```python
from build123d import *

# Parameters (mm, degrees)
F0_W      = 121.92
F0_H      = 71.12
F1_DEPTH  = 35.56
F2_W      = 3.81
F2_H      = 3.81
F3_DEPTH  = 12.7
F4_W      = 69.85
F4_H      = 47.625
F5_DEPTH  = 15.24
F6_W      = 27.94
F6_H      = 6.35
F7_DEPTH  = 71.12
F8_W      = 15.24
F8_H      = 6.35
F9_DEPTH  = 121.92
F10_W     = 27.94
F10_H     = 15.24
F11_DEPTH = 15.24
F12_DEPTH = 35.561
F13_W     = 40.005
F13_H     = 6.6675
F14_DEPTH = 35.561
F15_W     = 40.005
F15_H     = 15.24
F16_DEPTH = 4.2690588161
F17_W     = 40.005
F17_H     = 15.24
F18_DEPTH = 4.0254006162
F19_W     = 20.955
F19_H     = 14.605
F20_DEPTH = 25.4
F21_W     = 14.605
F21_H     = 15.24
F22_DEPTH = 17.6893454045
F23_W     = 14.605
F23_H     = 15.24
F24_DEPTH = 16.1260850728
F25_W     = 20.955
F25_H     = 15.24
F26_DEPTH = 12.7
F27_W     = 6.6675
F27_H     = 15.24
F28_DEPTH = 25.4
F29_W     = 6.6675
F29_H     = 15.24
F30_DEPTH = 25.4
F31_W     = 20.955
F31_H     = 15.24
F32_DEPTH = 12.7


with BuildPart() as f1:
    # F0 (on Top) → F1 (new body)
    with BuildSketch(Plane.XY):
        Rectangle(F0_W, F0_H)
    extrude(amount=F1_DEPTH)

    # F2 (on Top) → F3 (cut)
    with BuildSketch(Plane.XY):
        Polygon((59.055, -19.685), (52.07, -19.685), (52.07, -22.86), (55.88, -22.86), (55.88, -30.48), (48.26, -30.48), (48.26, -26.67), (45.085, -26.67), (45.085, -33.655), (59.055, -33.655), align=None)
        Polygon((52.07, -22.86), (52.07, -19.685), (45.085, -19.685), (45.085, -26.67), (48.26, -26.67), (48.26, -22.86), align=None)
        with Locations((50.165, -24.765)):
            Rectangle(F2_W, F2_H)
        Polygon((55.88, -22.86), (52.07, -22.86), (52.07, -26.67), (48.26, -26.67), (48.26, -30.48), (55.88, -30.48), align=None)
        Polygon((45.085, 33.655), (45.085, 26.67), (48.26, 26.67), (48.26, 30.48), (55.88, 30.48), (55.88, 22.86), (52.07, 22.86), (52.07, 19.685), (59.055, 19.685), (59.055, 33.655), align=None)
        Polygon((48.26, 26.67), (45.085, 26.67), (45.085, 19.685), (52.07, 19.685), (52.07, 22.86), (48.26, 22.86), align=None)
        Polygon((48.26, 30.48), (48.26, 26.67), (52.07, 26.67), (52.07, 22.86), (55.88, 22.86), (55.88, 30.48), align=None)
        with Locations((50.165, 24.765)):
            Rectangle(F2_W, F2_H)
        Polygon((-45.085, 26.67), (-48.26, 26.67), (-48.26, 22.86), (-52.07, 22.86), (-52.07, 19.685), (-45.085, 19.685), align=None)
        Polygon((-52.07, 22.86), (-52.07, 26.67), (-48.26, 26.67), (-48.26, 30.48), (-55.88, 30.48), (-55.88, 22.86), align=None)
        Polygon((-48.26, 30.48), (-48.26, 26.67), (-45.085, 26.67), (-45.085, 33.655), (-59.055, 33.655), (-59.055, 19.685), (-52.07, 19.685), (-52.07, 22.86), (-55.88, 22.86), (-55.88, 30.48), align=None)
        with Locations((-50.165, 24.765)):
            Rectangle(F2_W, F2_H)
        Polygon((-52.07, -22.86), (-52.07, -19.685), (-59.055, -19.685), (-59.055, -33.655), (-45.085, -33.655), (-45.085, -26.67), (-48.26, -26.67), (-48.26, -30.48), (-55.88, -30.48), (-55.88, -22.86), align=None)
        Polygon((-52.07, -26.67), (-52.07, -22.86), (-55.88, -22.86), (-55.88, -30.48), (-48.26, -30.48), (-48.26, -26.67), align=None)
        with Locations((-50.165, -24.765)):
            Rectangle(F2_W, F2_H)
        Polygon((-45.085, -19.685), (-52.07, -19.685), (-52.07, -22.86), (-48.26, -22.86), (-48.26, -26.67), (-45.085, -26.67), align=None)
    extrude(amount=F3_DEPTH, mode=Mode.SUBTRACT)

    # F4 (on face) → F5 (cut)
    with BuildSketch(Plane(origin=(0, 0, 0), x_dir=(1, 0, 0), z_dir=(0, 0, -1))):
        Rectangle(F4_W, F4_H)
    extrude(amount=-F5_DEPTH, mode=Mode.SUBTRACT)

    # F6 (on face) → F7 (cut, through all)
    with BuildSketch(Plane.XZ.offset(35.56)):
        with Locations((-44.45, 29.845)):
            Rectangle(F6_W, F6_H)
        with Locations((-16.51, 29.845)):
            Rectangle(F6_W, F6_H)
        with Locations((-16.51, 23.495)):
            Rectangle(F6_W, F6_H)
        with Locations((-44.45, 23.495)):
            Rectangle(F6_W, F6_H)
        with Locations((16.51, 29.845)):
            Rectangle(F6_W, F6_H)
        with Locations((16.51, 23.495)):
            Rectangle(F6_W, F6_H)
        with Locations((44.45, 29.845)):
            Rectangle(F6_W, F6_H)
        with Locations((44.45, 23.495)):
            Rectangle(F6_W, F6_H)
    extrude(amount=-F7_DEPTH, mode=Mode.SUBTRACT)

    # F8 (on face) → F9 (cut, through all)
    with BuildSketch(Plane(origin=(-60.96, 0, 0), x_dir=(0, -1, 0), z_dir=(-1, 0, 0))):
        with Locations((-25.4, 29.845)):
            Rectangle(F8_W, F8_H)
        with Locations((-10.16, 29.845)):
            Rectangle(F8_W, F8_H)
        with Locations((-10.16, 23.495)):
            Rectangle(F8_W, F8_H)
        with Locations((-25.4, 23.495)):
            Rectangle(F8_W, F8_H)
        with Locations((10.16, 23.495)):
            Rectangle(F8_W, F8_H)
        with Locations((10.16, 29.845)):
            Rectangle(F8_W, F8_H)
        with Locations((25.4, 29.845)):
            Rectangle(F8_W, F8_H)
        with Locations((25.4, 23.495)):
            Rectangle(F8_W, F8_H)
    extrude(amount=-F9_DEPTH, mode=Mode.SUBTRACT)

    # F10 (on face) → F11 (cut, through all)
    with BuildSketch(Plane.XY.offset(35.56)):
        with Locations((-44.45, 25.4)):
            Rectangle(F10_W, F10_H)
        with Locations((-16.51, 25.4)):
            Rectangle(F10_W, F10_H)
        with Locations((-16.51, 10.16)):
            Rectangle(F10_W, F10_H)
        with Locations((-44.45, 10.16)):
            Rectangle(F10_W, F10_H)
        with Locations((16.51, 25.4)):
            Rectangle(F10_W, F10_H)
        with Locations((16.51, 10.16)):
            Rectangle(F10_W, F10_H)
        with Locations((44.45, 25.4)):
            Rectangle(F10_W, F10_H)
        with Locations((44.45, 10.16)):
            Rectangle(F10_W, F10_H)
        with Locations((-44.45, -10.16)):
            Rectangle(F10_W, F10_H)
        with Locations((-16.51, -10.16)):
            Rectangle(F10_W, F10_H)
        with Locations((-16.51, -25.4)):
            Rectangle(F10_W, F10_H)
        with Locations((-44.45, -25.4)):
            Rectangle(F10_W, F10_H)
        with Locations((16.51, -25.4)):
            Rectangle(F10_W, F10_H)
        with Locations((16.51, -10.16)):
            Rectangle(F10_W, F10_H)
        with Locations((44.45, -25.4)):
            Rectangle(F10_W, F10_H)
        with Locations((44.45, -10.16)):
            Rectangle(F10_W, F10_H)
    extrude(amount=-F11_DEPTH, mode=Mode.SUBTRACT)

    # F2 (on Top) → F12 (cut, through all)
    with BuildSketch(Plane.XY):
        with Locations((50.165, -24.765)):
            Rectangle(F2_W, F2_H)
        Polygon((55.88, -22.86), (52.07, -22.86), (52.07, -26.67), (48.26, -26.67), (48.26, -30.48), (55.88, -30.48), align=None)
        with Locations((50.165, 24.765)):
            Rectangle(F2_W, F2_H)
        Polygon((48.26, 30.48), (48.26, 26.67), (52.07, 26.67), (52.07, 22.86), (55.88, 22.86), (55.88, 30.48), align=None)
        Polygon((-52.07, 22.86), (-52.07, 26.67), (-48.26, 26.67), (-48.26, 30.48), (-55.88, 30.48), (-55.88, 22.86), align=None)
        with Locations((-50.165, 24.765)):
            Rectangle(F2_W, F2_H)
        Polygon((-52.07, -26.67), (-52.07, -22.86), (-55.88, -22.86), (-55.88, -30.48), (-48.26, -30.48), (-48.26, -26.67), align=None)
        with Locations((-50.165, -24.765)):
            Rectangle(F2_W, F2_H)
    extrude(amount=F12_DEPTH, mode=Mode.SUBTRACT)

    # F13 (on face) → F14 (cut, through all)
    with BuildSketch(Plane(origin=(0, 0, 0), x_dir=(1, 0, 0), z_dir=(0, 0, -1))):
        with Locations((22.5425, 29.68625)):
            Rectangle(F13_W, F13_H)
        with Locations((-22.5425, 29.68625)):
            Rectangle(F13_W, F13_H)
        with Locations((22.5425, -29.68625)):
            Rectangle(F13_W, F13_H)
        with Locations((-22.5425, -29.68625)):
            Rectangle(F13_W, F13_H)
    extrude(amount=-F14_DEPTH, mode=Mode.SUBTRACT)

    # F15 (on face) → F16 (cut)
    with BuildSketch(Plane.XZ.offset(35.56)):
        with Locations((22.5425, 10.16)):
            Rectangle(F15_W, F15_H)
        with Locations((-22.5425, 10.16)):
            Rectangle(F15_W, F15_H)
    extrude(amount=-F16_DEPTH, mode=Mode.SUBTRACT)

    # F17 (on face) → F18 (cut)
    with BuildSketch(Plane(origin=(0, 35.56, 0), x_dir=(-1, 0, 0), z_dir=(0, 1, 0))):
        with Locations((22.5425, 10.16)):
            Rectangle(F17_W, F17_H)
        with Locations((-22.5425, 10.16)):
            Rectangle(F17_W, F17_H)
    extrude(amount=-F18_DEPTH, mode=Mode.SUBTRACT)

    # F19 (on face) → F20 (cut)
    with BuildSketch(Plane(origin=(0, 0, 0), x_dir=(1, 0, 0), z_dir=(0, 0, -1))):
        with Locations((47.9425, 9.8425)):
            Rectangle(F19_W, F19_H)
        with Locations((-47.9425, -9.8425)):
            Rectangle(F19_W, F19_H)
        with Locations((47.9425, -9.8425)):
            Rectangle(F19_W, F19_H)
        with Locations((-47.9425, 9.8425)):
            Rectangle(F19_W, F19_H)
    extrude(amount=-F20_DEPTH, mode=Mode.SUBTRACT)

    # F21 (on face) → F22 (cut)
    with BuildSketch(Plane.YZ.offset(60.96)):
        with Locations((9.8425, 10.16)):
            Rectangle(F21_W, F21_H)
        with Locations((-9.8425, 10.16)):
            Rectangle(F21_W, F21_H)
    extrude(amount=-F22_DEPTH, mode=Mode.SUBTRACT)

    # F23 (on face) → F24 (cut)
    with BuildSketch(Plane(origin=(-60.96, 0, 0), x_dir=(0, -1, 0), z_dir=(-1, 0, 0))):
        with Locations((-9.8425, 10.16)):
            Rectangle(F23_W, F23_H)
        with Locations((9.8425, 10.16)):
            Rectangle(F23_W, F23_H)
    extrude(amount=-F24_DEPTH, mode=Mode.SUBTRACT)

    # F25 (on face) → F26 (cut)
    with BuildSketch(Plane.XZ.offset(2.54)):
        with Locations((47.9425, 10.16)):
            Rectangle(F25_W, F25_H)
    extrude(amount=-F26_DEPTH, mode=Mode.SUBTRACT)

    # F27 (on face) → F28 (cut)
    with BuildSketch(Plane.YZ.offset(2.54)):
        with Locations((-29.68625, 10.16)):
            Rectangle(F27_W, F27_H)
    extrude(amount=-F28_DEPTH, mode=Mode.SUBTRACT)

    # F29 (on face) → F30 (cut)
    with BuildSketch(Plane.YZ.offset(2.54)):
        with Locations((29.68625, 10.16)):
            Rectangle(F29_W, F29_H)
    extrude(amount=-F30_DEPTH, mode=Mode.SUBTRACT)

    # F31 (on face) → F32 (cut)
    with BuildSketch(Plane(origin=(0, 2.54, 0), x_dir=(-1, 0, 0), z_dir=(0, 1, 0))):
        with Locations((47.9425, 10.16)):
            Rectangle(F31_W, F31_H)
    extrude(amount=-F32_DEPTH, mode=Mode.SUBTRACT)


solid = f1.part
```
Geometry: final body of the model. Coordinates: model frame, mm. A direction names the side the tool comes from. Coordinates: 2 decimals unless noted, no trailing zeros. Write each loop counter-clockwise with the first axis right and the second up, starting at its lowest first coordinate (ties: lowest second). Pieces come first, ordered by that corner, then holes. Notation, with made-up numbers: M 62,-8 L 101,-8 A14 ccw 101,0 Z; hole C 13,70.25 d1. An arc over 180 degrees is marked long. Answer as CSV lines item,"result". Start each with the question number.
Q1. Cut plane C-C on z = 31.5. Count the separate pieces of the cut face and the enclosed holes in it, then the cut area to 3 significant figures.
Q2. Cut plane B-B on y = 21. Return the cut outline in (x, z) (3 decimals).
Q3. Reachability of faces 3 (the flat face through (-2.54, -34, 10)), 4 (the flat face through (0, 2.54, 27)), 5 (the flat face through (58.42, -10, 19)), 6 (the flat face through (0, -23.812, 8)), 7 (the flat face through (-2.54, 18, 34)) from +Z, -Z, +X, -X, +Y, -Y: full face, straight path, thin tool, end or side. Return the list, or none.
Q4. Pin query (flat end, axial travel): P1, Ø6, axis at x = 16, z = 30.5, coming from the -Y side; P2, Ø1.5, axis at x = 17, y = -15, coming from the +Z side; P3, Ø2, axis at x = 6, z = 15.5, coming from the +Y side. Return the tip coordinate at first contact, or that it passes through.
Q5. Line query: line 1 (X direction, y = 1.5, z = 29.5); line 2 (X direction, y = -26.5, z = 19) (3 decimals); line 3 (X direction, y = -24, z = 6) (3 decimals). Output: solid intervals per line, ascending. Write a range as from..to.
Q6. Mould query, pull axis Y, two halves, no side actions, for faces 1 (the flat face through (58.42, 0, 27)), 2 (the flat face through (58.42, -10, 1)). Classes: released by +Y, released by -Y, zero draft, split by the parting line, or undercut.
Q7. Cut plane A-A on x = 1. Return the cut outline in (y, z), then the cut area to 3 significant figures.
Findings below:
1,separate pieces,"9"
1,enclosed holes,"0"
1,area,"103 mm2"
2,outline,"M -60.96,0 L -59.055,0 L -59.055,12.7 L -45.085,12.7 L -45.085,0 L -34.925,0 L -34.925,15.24 L 34.925,15.24 L 34.925,0 L 45.085,0 L 45.085,12.7 L 59.055,12.7 L 59.055,0 L 60.96,0 L 60.96,20.32 L -60.96,20.32 Z; M -60.96,33.02 L -58.42,33.02 L -58.42,35.56 L -60.96,35.56 Z; M -2.54,33.02 L 2.54,33.02 L 2.54,35.56 L -2.54,35.56 Z; M 58.42,33.02 L 60.96,33.02 L 60.96,35.56 L 58.42,35.56 Z"
3,face 3,"-Y"
3,face 4,"+X, -X"
3,face 5,"+Z, -Z"
3,face 6,"-Z"
3,face 7,"+Z"
4,P1,"stops at y = -35.56"
4,P2,"stops at z = 20.32"
4,P3,"stops at y = 26.35"
5,line 1,"x = -60.96..-58.42, -2.54..2.54, 58.42..60.96"
5,line 2,"x = -60.96..-55.88, -48.26..-42.545, -2.54..2.54, 42.545..48.26, 55.88..60.96"
5,line 3,"x = -60.96..-59.055, -45.085..45.085, 59.055..60.96"
6,face 1,"zero draft"
6,face 2,"undercut"
7,outline,"M -35.56,0 L -23.81,0 L -23.81,15.24 L 23.81,15.24 L 23.81,0 L 35.56,0 L 35.56,35.56 L -35.56,35.56 Z; hole M -33.02,2.54 L -26.35,2.54 L -26.35,17.78 L -33.02,17.78 Z; hole M -33.02,20.32 L -2.54,20.32 L -2.54,33.02 L -33.02,33.02 Z; hole M 2.54,20.32 L 33.02,20.32 L 33.02,33.02 L 2.54,33.02 Z; hole M 26.35,2.54 L 33.02,2.54 L 33.02,17.78 L 26.35,17.78 Z"
7,area,"826 mm2"
